Check sheet for the drawn part. Datum: minimum x, y, z corner. Units: mm. A direction names the side the tool comes from. Coordinates: 2 decimals unless noted, no trailing zeros. Loops run counter-clockwise (first coordinate to the right, second up) from the corner with the lowest first, then second, coordinate; pieces in that order, holes last.
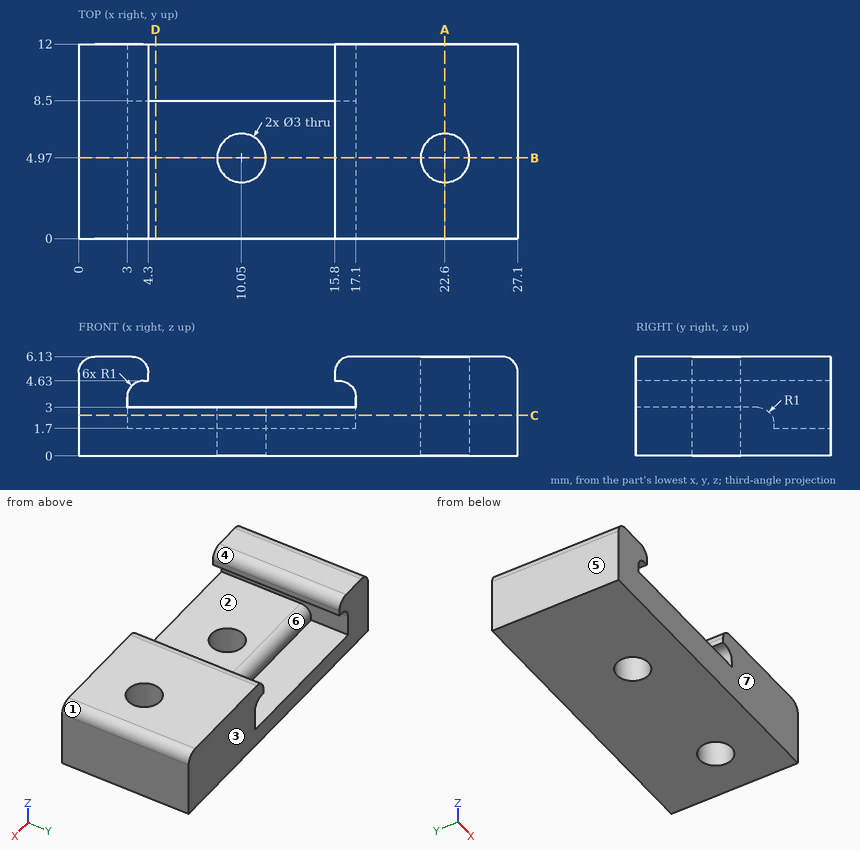
(1) Sectioned sample at A-A on x = 22.6. Record the cut outline in (y, z), and give its area (3 significant figures).
Findings:
outline: (0, 0) - (3.47, 0) - (3.47, 6.13) - (0, 6.13) - close; (6.47, 0) - (12, 0) - (12, 6.13) - (6.47, 6.13) - close
area: 55.2 mm2
(2) Sectioned sample at B-B on y = 4.97. Record the cut outline in (x, z), and give its area (3 significant figures).
Findings:
outline: (0, 0) - (8.55, 0) - (8.55, 3) - (3, 3) - (3, 3.63) arc R1 cw to (4, 4.63) - (4.3, 4.63) - (4.3, 5.13) arc R1 ccw to (3.3, 6.13) - (1, 6.13) arc R1 ccw to (0, 5.13) - close; (11.55, 0) - (21.1, 0) - (21.1, 6.13) - (16.8, 6.13) arc R1 ccw to (15.8, 5.13) - (15.8, 4.63) - (16.1, 4.63) arc R1 cw to (17.1, 3.63) - (17.1, 3) - (11.55, 3) - close; (24.1, 0) - (27.1, 0) - (27.1, 5.13) arc R1 ccw to (26.1, 6.13) - (24.1, 6.13) - close
area: 98.1 mm2
(3) Sectioned sample at D-D on x = 4.75. Record the cut outline in (y, z).
Findings:
outline: (0, 0) - (12, 0) - (12, 1.7) - (8.5, 1.7) - (8.5, 2) arc R1 ccw to (7.5, 3) - (0, 3) - close
(4) Sectioned sample at C-C on z = 2.5. Record the cut outline in (x, y), and give its area (3 significant figures).
Findings:
outline: (0, 0) - (27.1, 0) - (27.1, 12) - (17.1, 12) - (17.1, 8.37) - (3, 8.37) - (3, 12) - (0, 12) - close; hole circle Ø3 at (10.05, 4.97); hole circle Ø3 at (22.6, 4.97)
area: 260 mm2
(5) Draft check along X on the marked faces 1, 2 and 3. Enter one of: +X half, -X half, draft (parallel to the pull), parting line (faces both ways), or undercut.
Findings:
face 1: +X half
face 2: undercut
face 3: draft
(6) Access from +Z, -Z, +X, -X, +Y, -Y to the whole of each face (thin tool, end or side, straight path). Record for the marked faces 4, 5, 6 and 7.
Findings:
face 4: +Z, +Y, -Y
face 5: +Z, -Z, -X, +Y, -Y
face 6: +Y
face 7: +Z, -Z, +X, -X, -Y
(7) Scan lines: L1, parallel to Y at x = 10.05, z = 0.85; L2, parallel to X at y = 11.25, z = 1.75; L3, parallel to X at y = 9, z = 4.25. Record each from-to range of solid material in increasing order.
Findings:
L1: y = 0 to 3.47, 6.47 to 12
L2: x = 0 to 3, 17.1 to 27.1
L3: x = 0 to 3.22, 16.88 to 27.1
(8) Gauge pin test, flat ends, axial feed: pin 1 Ø1.5 at (x, y) = (5.5, 4) entering from +Z; pin 2 Ø2 at (y, z) = (5.5, 3) entering from -X. Record the tip position at first contact, or that the pin passes through.
Findings:
pin 1: stops at z = 3
pin 2: stops at x = 0
